Geometry check sheet. Reference: drawing and pictorial views, mm from the part's lowest x, y, z. A direction names the side the tool comes from. Give positions to 0.01 mm unless a question says otherwise; leave off trailing zeros. Loops run counter-clockwise (first coordinate to the right, second up) from the corner with the lowest first, then second, coordinate; pieces in that order, holes last. Notation, with made-up numbers: (-37.5, 50.25) -> (19.5, 50.25) arc R24 ccw to (19.5, 75.25) -> close; hole circle Ø9 at (82, 1.25). An arc over 180 degrees is marked (long way). Answer in a Markdown table with one row per item. Add a question column.
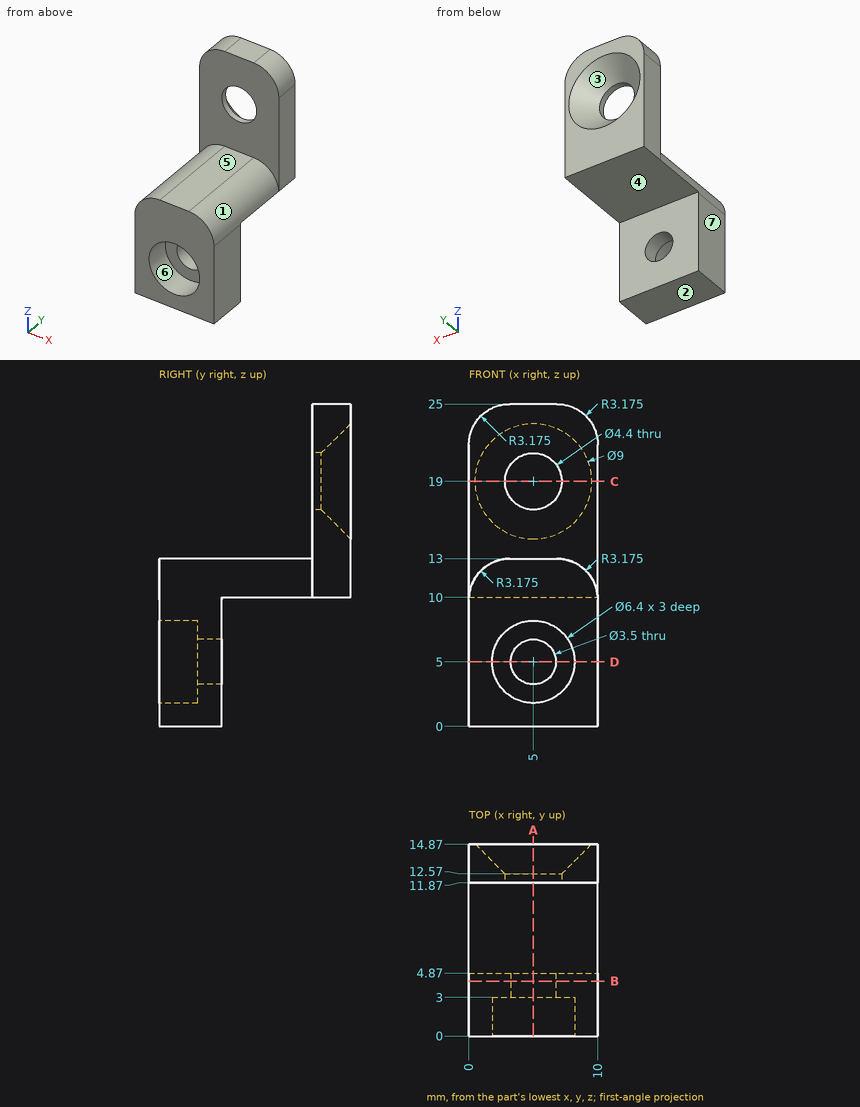
1. Gauge pin test, flat ends, axial feed: pin 1 Ø4 at (x, z) = (5, 5) entering from -Y; pin 2 Ø4 at (x, y) = (5, 7) entering from +Z; pin 3 Ø1.5 at (y, z) = (9.5, 12.5) entering from +X. Record the tip position at first contact, or that the pin passes through.
2. Sectioned sample at C-C (z = 19). Enter the section's corners in (x, y), plus the area to 3 significant figures.
3. Release check for a two-part mould opening along Z. For the marked faces 1, 2 and 3 record: released by +Z, released by -Z, zero draft, split by the parting line, or undercut.
4. Access from +Z, -Z, +X, -X, +Y, -Y to the whole of each face (thin tool, end or side, straight path). Record for the marked faces 4, 5, 6 and 7.
5. Sectioned sample at D-D (z = 5). Enter the section's corners in (x, y), plus the area to 3 significant figures.
6. Material ranges on L1, parallel to X at y = 12.3, z = 19; L2, parallel to X at y = 2.4, z = 5; L3, parallel to Z at x = 5, y = 1.8, recorded low to high. Write a range as from..to.
7. Sectioned sample at A-A (x = 5). Enter the section's corners in (y, z).
8. Sectioned sample at B-B (y = 4.25). Enter the section's corners in (x, z) (3 decimals), plus the area to 3 significant figures.
Response:
| question | item | result |
|---|---|---|
| 1 | pin 1 | stops at y = 3 |
| 1 | pin 2 | stops at z = 13 |
| 1 | pin 3 | stops at x = 9.35 |
| 2 | outline | (0, 11.87) -> (2.8, 11.87) -> (2.8, 12.57) -> (0.5, 14.87) -> (0, 14.87) -> close; (7.2, 11.87) -> (10, 11.87) -> (10, 14.87) -> (9.5, 14.87) -> (7.2, 12.57) -> close |
| 2 | area | 11.5 mm2 |
| 3 | face 1 | released by +Z |
| 3 | face 2 | released by -Z |
| 3 | face 3 | undercut |
| 4 | face 4 | -Z, +X, -X, +Y |
| 4 | face 5 | +Z, +X, -X, -Y |
| 4 | face 6 | -Y |
| 4 | face 7 | +Z, -Z, -X, +Y, -Y |
| 5 | outline | (0, 0) -> (1.8, 0) -> (1.8, 3) -> (3.25, 3) -> (3.25, 4.87) -> (0, 4.87) -> close; (6.75, 3) -> (8.2, 3) -> (8.2, 0) -> (10, 0) -> (10, 4.87) -> (6.75, 4.87) -> close |
| 5 | area | 23.0 mm2 |
| 6 | L1 | x = 0..2.8, 7.2..10 |
| 6 | L2 | x = 0..1.8, 8.2..10 |
| 6 | L3 | z = 0..1.8, 8.2..13 |
| 7 | outline | (0, 0) -> (4.87, 0) -> (4.87, 3.25) -> (3, 3.25) -> (3, 1.8) -> (0, 1.8) -> close; (0, 8.2) -> (3, 8.2) -> (3, 6.75) -> (4.87, 6.75) -> (4.87, 10) -> (14.87, 10) -> (14.87, 14.5) -> (12.57, 16.8) -> (11.87, 16.8) -> (11.87, 13) -> (0, 13) -> close; (11.87, 21.2) -> (12.57, 21.2) -> (14.87, 23.5) -> (14.87, 25) -> (11.87, 25) -> close |
| 8 | outline | (0, 0) -> (10, 0) -> (10, 9.825) arc R3.175 ccw to (6.825, 13) -> (3.175, 13) arc R3.175 ccw to (0, 9.825) -> close; hole circle Ø3.5 at (5, 5) |
| 8 | area | 116 mm2 |
